Could you check a few things on this drawing? It's one solid part, dimensions in mm from its lowest x, y, z. Round coordinates to 2 decimals unless told otherwise and drop trailing zeros. Order: outer loops, then holes, each group sorted by start corner. A loop starts at its lowest first (then second) coordinate and runs counter-clockwise, first axis right, second up.
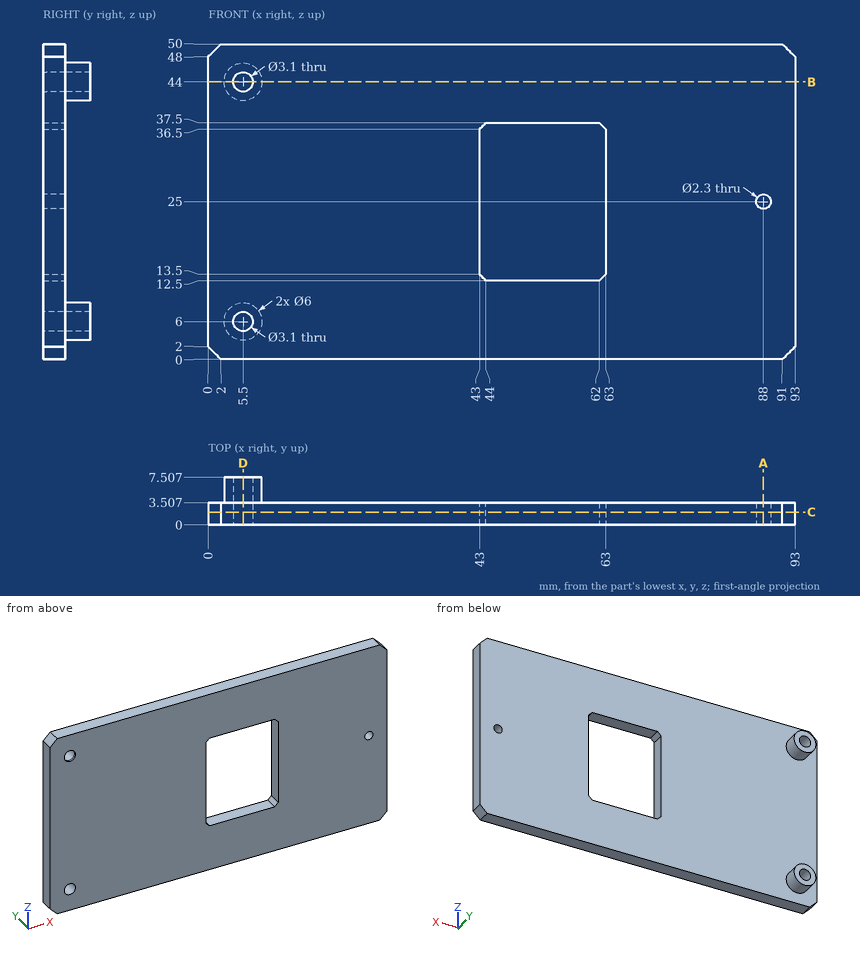
(1) I'm going to push flat-ended pins straight in: pin 1 Ø3 at (x, z) = (13, 27.5) entering from -Y; pin 2 Ø3 at (x, z) = (5.5, 6) entering from +Y; pin 3 Ø2 at (y, z) = (5.5, 9) entering from -X (1 decimal). Where does each tip first touch, or does it pass through?
(2) I want a section at D-D, the plane x = 5.5. List the corners of the cut face in (y, z) for me, plus the area to 3 significant figures.
(3) I want a section at A-A, the plane x = 88. List the corners of the cut face in (y, z) for me, plus the area to 3 significant figures.
(4) I want a section at C-C, the plane y = 2. List the corners of the cut face in (x, z) for me.
(5) Please list where these lines run through material, in increasing order: probe 1 along Z at (x, y) = (5.5, 0.25); probe 2 along X at (y, z) = (1.6, 25); probe 3 along X at (y, z) = (2, 14).
(6) I want a section at B-B, the plane z = 44. List the corners of the cut face in (x, y) for me, plus the area to 3 significant figures.
Ans:
1. pin 1: stops at y = 0
1. pin 2: passes through
1. pin 3: stops at x = 3.3
2. outline: (0, 0) - (3.51, 0) - (3.51, 3) - (7.51, 3) - (7.51, 4.45) - (0, 4.45) - close; (0, 7.55) - (7.51, 7.55) - (7.51, 9) - (3.51, 9) - (3.51, 41) - (7.51, 41) - (7.51, 42.45) - (0, 42.45) - close; (0, 45.55) - (7.51, 45.55) - (7.51, 47) - (3.51, 47) - (3.51, 50) - (0, 50) - close
2. area: 177 mm2
3. outline: (0, 0) - (3.51, 0) - (3.51, 23.85) - (0, 23.85) - close; (0, 26.15) - (3.51, 26.15) - (3.51, 50) - (0, 50) - close
3. area: 167 mm2
4. outline: (0, 2) - (2, 0) - (91, 0) - (93, 2) - (93, 48) - (91, 50) - (2, 50) - (0, 48) - close; hole circle Ø3.1 at (5.5, 6); hole circle Ø3.1 at (5.5, 44); hole (43, 13.5) - (44, 12.5) - (62, 12.5) - (63, 13.5) - (63, 36.5) - (62, 37.5) - (44, 37.5) - (43, 36.5) - close; hole circle Ø2.3 at (88, 25)
5. probe 1: z = 0 to 4.45, 7.55 to 42.45, 45.55 to 50
5. probe 2: x = 0 to 43, 63 to 86.85, 89.15 to 93
5. probe 3: x = 0 to 43, 63 to 93
6. outline: (0, 0) - (3.95, 0) - (3.95, 7.51) - (2.5, 7.51) - (2.5, 3.51) - (0, 3.51) - close; (7.05, 0) - (93, 0) - (93, 3.51) - (8.5, 3.51) - (8.5, 7.51) - (7.05, 7.51) - close
6. area: 327 mm2
